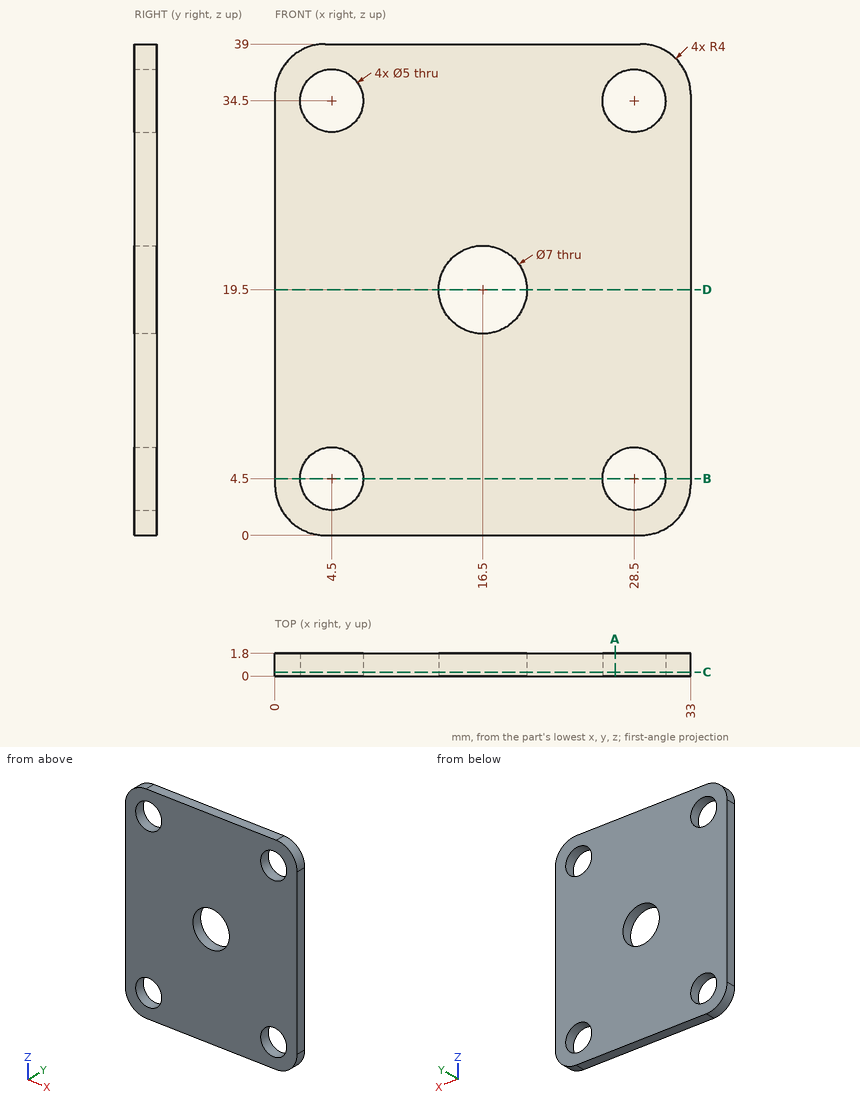
The figure shows three views and two pictorial views of one solid part (mm, origin at its lowest corner). Answer the questions. Give positions to 0.01 mm unless a question says otherwise; leave off trailing zeros. Order: outer loops, then holes, each group sorted by start corner. A loop starts at its lowest first (then second) coordinate and runs counter-clockwise, first axis right, second up. Notation, with made-up numbers: (0, 46.5) -> (54, 46.5) arc R30 ccw to (54, 72.5) -> close; hole circle Ø10 at (-13, -2.75). An arc over 180 degrees is marked (long way). One line per item, written item: value.
1) Find section C-C, the plane y = 0.3. Determine the outline of the cut face in (x, z), plus the area to 3 significant figures.
Reported:
outline: (0, 4) arc R4 ccw to (4, 0) -> (29, 0) arc R4 ccw to (33, 4) -> (33, 35) arc R4 ccw to (29, 39) -> (4, 39) arc R4 ccw to (0, 35) -> close; hole circle Ø5 at (4.5, 4.5); hole circle Ø5 at (4.5, 34.5); hole circle Ø7 at (16.5, 19.5); hole circle Ø5 at (28.5, 4.5); hole circle Ø5 at (28.5, 34.5)
area: 1,160 mm^2
2) Find section A-A, the plane x = 27. Determine the outline of the cut face in (y, z), plus the area to 3 significant figures.
Reported:
outline: (0, 0) -> (1.8, 0) -> (1.8, 2.5) -> (0, 2.5) -> close; (0, 6.5) -> (1.8, 6.5) -> (1.8, 32.5) -> (0, 32.5) -> close; (0, 36.5) -> (1.8, 36.5) -> (1.8, 39) -> (0, 39) -> close
area: 55.8 mm^2
3) Find section B-B, the plane z = 4.5. Determine the outline of the cut face in (x, y).
Reported:
outline: (0, 0) -> (2, 0) -> (2, 1.8) -> (0, 1.8) -> close; (7, 0) -> (26, 0) -> (26, 1.8) -> (7, 1.8) -> close; (31, 0) -> (33, 0) -> (33, 1.8) -> (31, 1.8) -> close
4) Find section D-D, the plane z = 19.5. Determine the outline of the cut face in (x, y), plus the area to 3 significant figures.
Reported:
outline: (0, 0) -> (13, 0) -> (13, 1.8) -> (0, 1.8) -> close; (20, 0) -> (33, 0) -> (33, 1.8) -> (20, 1.8) -> close
area: 46.8 mm^2
5) Find the intervals of material crossed by line 1 (X direction, y = 0.65, z = 34.5); line 2 (X direction, y = 0.95, z = 36.5); line 3 (Z direction, x = 30.5, y = 1.15), in increasing order.
Reported:
line 1: x = 0 to 2, 7 to 26, 31 to 33
line 2: x = 0.29 to 3, 6 to 27, 30 to 32.71
line 3: z = 0.29 to 3, 6 to 33, 36 to 38.71
6) Flat-ended cylindrical pins translate along their axes: P1, Ø3, axis at x = 11.5, z = 5, coming from the -Y side; P2, Ø5.5, axis at x = 16.5, z = 19.5, coming from the +Y side. Find the tip coordinate at first contact, or state that the pin passes through.
Reported:
P1: stops at y = 0
P2: passes through
